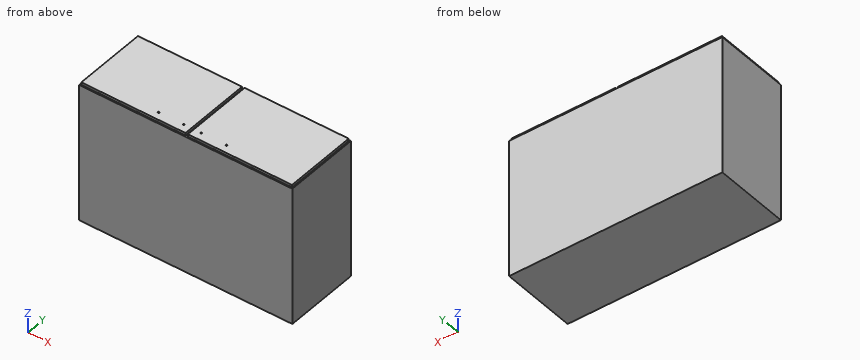
Autodesk Inventor part; units mm, degrees
ref_plane "Plano de trabajo1" through (-24.9992, 73.6009, 295.6345) normal (0, 1, 0) x (1, 0, 0)
ref_plane "YZ Plane" through (0, 0, 0) normal (1, 0, 0) x (0, 1, 0)
ref_plane "XZ Plane" through (0, 0, 0) normal (0, 1, 0) x (-1, 0, 0)
ref_plane "Plano de trabajo1" through (-24.9992, 73.6009, 295.6345) normal (0, 1, 0) x (1, 0, 0)
sketch "Boceto1" plane through (-24.9992, 73.6009, 295.6345) normal (0, 1, 0) x (1, 0, 0)
  line L0 (0, -21.25) -> (0, -5.817)
  line L1 (0, -21.25) -> (850, -21.25)
  line L2 (850, -21.25) -> (850, 528.929)
  line L3 (850, 528.929) -> (0, 528.929)
  line L4 (0, 528.929) -> (0, -21.25)
  point P0 (24.9992, 295.6345)
extrude "Extrusión1" add sketch "Boceto1" along normal blind 302.519
sketch "Boceto2" plane through (-24.9992, 73.6009, 316.8845) normal (0, 0, 1) x (1, 0, 0)
  line L0 (0, 0) -> (850, 0)
  line L1 (0, 0) -> (10, 0)
  line L2 (10, 0) -> (10, 10)
  line L3 (0, 302.519) -> (850, 302.519)
  line L4 (850, 302.519) -> (840, 302.519)
  line L5 (840, 302.519) -> (840, 292.519)
  line L6 (10, 10) -> (840, 10)
  line L7 (840, 10) -> (840, 292.519)
  line L8 (840, 292.519) -> (10, 292.519)
  line L9 (10, 292.519) -> (10, 10)
  point P0 (24.9992, -73.6009)
  dimension "espesor" = 10
  dimension "d3" = 10
  dimension "d4" = 10
  dimension "d5" = 10
extrude "Extrusión2" cut sketch "Boceto2" against normal blind 545
sketch "Boceto3" plane through (-24.9992, 73.6009, 316.8845) normal (0, 0, 1) x (1, 0, 0)
  line L0 (0, 0) -> (5, 0)
  line L1 (850, 0) -> (0, 0)
  line L2 (5, 0) -> (5, 5)
  line L3 (0, 302.519) -> (850, 302.519)
  line L4 (425, 302.519) -> (420, 302.519)
  line L5 (420, 302.519) -> (420, 297.519)
  line L6 (420, 297.519) -> (5, 297.519)
  line L7 (5, 297.519) -> (5, 5)
  line L8 (5, 5) -> (420, 5)
  line L9 (420, 5) -> (420, 297.519)
  line L10 (425, 302.519) -> (425, 0)
  line L11 (430, 297.519) -> (845, 297.519)
  line L12 (845, 297.519) -> (845, 5)
  line L13 (845, 5) -> (430, 5)
  line L14 (430, 5) -> (430, 297.519)
  point P0 (24.9992, -73.6009)
  dimension "d8" = 5
  dimension "d9" = 5
  dimension "d10" = 5
  dimension "d11" = 5
extrude "Extrusión3" add sketch "Boceto3" along normal blind 10 contours L7 L6 L9 L8 | L11 L12 L13 L14
sketch "Boceto4" plane through (-24.9992, 73.6009, 326.8845) normal (0, 0, 1) x (1, 0, 0)
  line L0 (5, 5) -> (420, 5)
  line L1 (420, 5) -> (420, 297.519)
  line L2 (420, 297.519) -> (5, 297.519)
  line L3 (5, 297.519) -> (5, 5)
  line L4 (845, 297.519) -> (430, 297.519)
  line L5 (430, 297.519) -> (430, 5)
  line L6 (430, 5) -> (845, 5)
  line L7 (845, 5) -> (845, 297.519)
  line L8 (10, 10) -> (10, 292.519)
  line L9 (10, 35.2519) -> (845, 35.2519) construction
  line L10 (340, 5) -> (340, 297.519) construction
  line L11 (430, 5) -> (845, 5)
  line L12 (510, 5) -> (510, 297.519) construction
  circle A0 centre (290, 35.2519) radius 3
  circle A1 centre (390, 35.2519) radius 3
  circle A2 centre (560, 35.2519) radius 3
  circle A3 centre (460, 35.2519) radius 3
  point P0 (24.9992, -73.6009)
  dimension "d15" = 30.2519
  dimension "d16" = 80
  dimension "d17" = 80
  dimension "d18" = 6
  dimension "d19" = 50
  dimension "d20" = 6
  dimension "d21" = 50
extrude "Extrusión4" cut sketch "Boceto4" against normal up to next contours A0 | A1 | A2 | A3
equation "\"d3\" = espesor"
equation "\"d4\" = espesor"
equation "\"d5\" = espesor"
equation "\"d8\" = 0.5 * espesor"
equation "\"d9\" = 0.5 * espesor"
equation "\"d10\" = 0.5 * espesor"
equation "\"d11\" = 0.5 * espesor"
equation "\"d12\" = espesor"
equation "\"d15\" = 0.1 * h_me"
properties part number "MuebleExtractor"
Input: part model. Units: mm. Frame: model coordinates. Coordinates: 2 decimals unless noted, no trailing zeros. Order: outer loops, then holes, each group sorted by start corner. A loop starts at its lowest first (then second) coordinate and runs counter-clockwise, first axis right, second up. Notation, with made-up numbers: M 51.25,86.5 L 76.25,86.5 A7 cw 76.25,99.5 Z; hole C 14.5,75.25 d6. An arc over 180 degrees is marked long. Write item = value, one per line. Start each with the question number.
(1) Section A-A on y = 243. Output: boundary loops of the cut face in (x, z).
(2) Line query: line 1 along Y through (x, z) = (137, -87); line 2 along Z through (x, y) = (309.5, 294.5); line 3 along X through (y, z) = (353, -128.5). Output: solid intervals per line, ascending. Write a range as [from, to].
(3) Section C-C on x = 115. Output: boundary loops of the cut face in (y, z), and give its area (3 significant figures).
(4) Section B-B on z = -74.5. Output: boundary loops of the cut face in (x, y), and give its area (3 significant figures).
(5) First-contact query: P1, Ø11, axis at x = 223, z = 324, coming from the -Y side; P2, Ø3, axis at x = 266, z = 321, coming from the +Y side; P3, Ø3, axis at y = 189, z = 321.5, coming from the +X side. Flat tips, straight axial feed; report the tip coordinate or a pass-through.
Result set:
q1.outline = M -25,-233.29 L 825,-233.29 L 825,316.88 L 820,316.88 L 820,326.88 L 405,326.88 L 405,316.88 L 815,316.88 L 815,-228.12 L -15,-228.12 L -15,316.88 L 395,316.88 L 395,326.88 L -20,326.88 L -20,316.88 L -25,316.88 Z
q2.line_1 = [73.6, 83.6], [366.12, 376.12]
q2.line_2 = [-233.29, -228.12], [316.88, 326.88]
q2.line_3 = [-25, -15], [815, 825]
q3.outline = M 73.6,-233.29 L 376.12,-233.29 L 376.12,316.88 L 371.12,316.88 L 371.12,326.88 L 78.6,326.88 L 78.6,316.88 L 73.6,316.88 Z; hole M 83.6,-228.12 L 366.12,-228.12 L 366.12,316.88 L 83.6,316.88 Z
q3.area = 15,400 mm²
q4.outline = M -25,73.6 L 825,73.6 L 825,376.12 L -25,376.12 Z; hole M -15,83.6 L 815,83.6 L 815,366.12 L -15,366.12 Z
q4.area = 22,700 mm²
q5.P1 = 78.6
q5.P2 = 371.12
q5.P3 = 820
